Part model, mm, in its own coordinate system. A direction names the side the tool comes from. Coordinates: 2 decimals unless noted, no trailing zeros. Loops run counter-clockwise (first coordinate to the right, second up) from the corner with the lowest first, then second, coordinate; pieces in that order, holes last. Notation, with made-up numbers: (75, -3.75) - (92, -3.75) arc R27 cw to (92, 14.25) - close; hole circle Ø3 at (78.25, -30.5). An arc over 180 degrees is marked (long way). Use a Markdown table: item, result. Add a question column.
1) Band-saw the part on D-D (z = 2.5). Give the cut face in (x, y), plus the area to 3 significant figures.
2) Drop flat-ended pins along their axis: P1, Ø0.8, axis at x = 0, y = -1.5, coming from the -Z side; P2, Ø5, axis at x = -4, y = -4, coming from the +Z side; P3, Ø5, axis at y = 4, z = 1.5, coming from the +X side. Give the stop position or say it passes through.
3) Pull direction X, two halves, no side cores. Call faces 1 (the face through (2, 0, 0)), 2 (the face through (0, 0, 2)), 3 (the face through (-3, 0, 6)): +X half, -X half, draft (parallel to the pull), parting line (faces both ways), or undercut.
4) Band-saw the part on C-C (z = 8). Give the cut face in (x, y), plus the area to 3 significant figures.
5) Band-saw the part on A-A (x = 0). Give the cut face in (y, z).
6) Band-saw the part on B-B (y = 0). Give the cut face in (x, z).
7) Probe probe 1 along X at (y, z) = (-0.5, 1.75); probe 2 along Y at (x, z) = (-0.5, 2.75); probe 3 along Z at (x, y) = (-0.25, -4.25). List the from-to ranges inside material, lowest first. Write a range as [from, to].
8) Tool access for faces 4 (the face through (-0.5, 0, 1)), 5 (the face through (2.4, -2.4, 3.5)), 6 (the face through (-1.19, -5.37, 2.08)): list every direction of +Z, -Z, +X, -X, +Y, -Y with a clear straight run to the whole face (end or side of a thin tool).
from build123d import *

# Parameters (mm, degrees)
ESQUISSE2_R             = 5.5
BOSS_EXTRU_1_DEPTH      = 3.5
ESQUISSE3_R             = 3
BOSS_EXTRU_2_DEPTH      = 6
CONG_2_R                = 0.7
CHANFREIN1_SIZE         = 0.5
ENL_V_MAT_EXTRU_1_DEPTH = 2


with BuildPart() as part:
    # Esquisse2 → Boss.-Extru.1 (new body)
    with BuildSketch(Plane.XY):
        Circle(ESQUISSE2_R)
    extrude(amount=BOSS_EXTRU_1_DEPTH)

    # Esquisse3 → Boss.-Extru.2 (add)
    with BuildSketch(Plane.XY.offset(3.5)):
        Circle(ESQUISSE3_R)
    extrude(amount=BOSS_EXTRU_2_DEPTH)

    # Congé2
    cong_2_edges = [part.edges().sort_by_distance(p)[0] for p in [
        (-5.5, 0, 0),
    ]]
    fillet(cong_2_edges, radius=CONG_2_R)

    # Chanfrein1
    chanfrein1_edges = [part.edges().sort_by_distance(p)[0] for p in [
        (-3, 0, 9.5),
    ]]
    chamfer(chanfrein1_edges, length=CHANFREIN1_SIZE)

    # Esquisse4 → Enlèv. mat.-Extru.1 (cut)
    with BuildSketch(Plane(origin=(0, 0, 0), x_dir=(-1, 0, 0), z_dir=(0, 0, -1))):
        with BuildLine():
            Line((-0.5, 5.477225575), (-0.5, -5.477225575))
            ThreePointArc((-0.5, -5.477225575), (0, -5.5), (0.5, -5.477225575))
            Line((0.5, -5.477225575), (0.5, 5.477225575))
            ThreePointArc((0.5, 5.477225575), (0, 5.5), (-0.5, 5.477225575))
        make_face()
    extrude(amount=-ENL_V_MAT_EXTRU_1_DEPTH, mode=Mode.SUBTRACT)


solid = part.part
Answer block:
| question | item | result |
|---|---|---|
| 1 | outline | circle Ø11 at (0, 0) |
| 1 | area | 95.0 mm2 |
| 2 | P1 | z = 2 |
| 2 | P2 | z = 3.5 |
| 2 | P3 | x = 5.29 |
| 3 | face 1 | draft |
| 3 | face 2 | undercut |
| 3 | face 3 | parting line |
| 4 | outline | circle Ø6 at (0, 0) |
| 4 | area | 28.3 mm2 |
| 5 | outline | (-5.5, 2) - (5.5, 2) - (5.5, 3.5) - (3, 3.5) - (3, 9) - (2.5, 9.5) - (-2.5, 9.5) - (-3, 9) - (-3, 3.5) - (-5.5, 3.5) - close |
| 6 | outline | (-5.5, 0.7) arc R0.7 ccw to (-4.8, 0) - (-0.5, 0) - (-0.5, 2) - (0.5, 2) - (0.5, 0) - (4.8, 0) arc R0.7 ccw to (5.5, 0.7) - (5.5, 3.5) - (3, 3.5) - (3, 9) - (2.5, 9.5) - (-2.5, 9.5) - (-3, 9) - (-3, 3.5) - (-5.5, 3.5) - close |
| 7 | probe 1 | [-5.48, -0.5], [0.5, 5.48] |
| 7 | probe 2 | [-5.48, 5.48] |
| 7 | probe 3 | [2, 3.5] |
| 8 | face 4 | -Z, +Y, -Y |
| 8 | face 5 | +Z |
| 8 | face 6 | +Z, -Z |
